The listing builds one solid part. Answer for the finished solid, in the listing's coordinates (mm). Face numbers are marked on the shaded views. A direction names the side the tool comes from. Give positions to 0.01 mm unless a question says otherwise; leave off trailing zeros. Write each loop counter-clockwise with the first axis right and the second up, starting at its lowest first coordinate (ties: lowest second). Pieces come first, ordered by that corner, then holes. Notation, with made-up numbers: (43.5, 28.5) -> (84.5, 28.5) arc R30 ccw to (84.5, 60.5) -> close; hole circle Ø5 at (-18, 10.5). An arc over 180 degrees is marked (long way). Put each result on its own line as item: value. Start each with the question number.
1) A cutting plane is placed at C-C (z = 3). Give the number of separate pieces and of enclosed holes in the cut face, then the cut area to 3 significant figures.
2) A cutting plane is placed at A-A (x = 4.5). Write down the section's boundary in (y, z).
3) A cutting plane is placed at B-B (x = 1.75). Write down the section's boundary in (y, z).
4) Find the intervals of material crossed by line 1 along Y through (x, z) = (4.5, 1.75); line 2 along Y through (x, z) = (5.25, 2); line 3 along Z through (x, y) = (1.25, 6), in increasing order. Write a range as from..to.
5) Flat-ended cylindrical pins translate along their axes: pin 1 Ø1.6 at (x, z) = (3, 5) entering from -Y; pin 2 Ø1 at (x, y) = (6, 3) entering from +Z. Find the tip coordinate at first contact, or state that the pin passes through.
6) For the marked faces 1 and 2, determine the directions among +Z, -Z, +X, -X, +Y, -Y from which every point of the face is accessible in a straight line to the end or side of a thin tool.
Autodesk Inventor part; units mm, degrees
ref_plane "YZ Plane" through (0, 0, 0) normal (1, 0, 0) x (0, 1, 0)
ref_plane "XZ Plane" through (0, 0, 0) normal (0, 1, 0) x (-1, 0, 0)
ref_plane "XY Plane" through (0, 0, 0) normal (0, 0, 1) x (1, 0, 0)
sketch "Skizze5" plane through (0, 0, 0) normal (1, 0, 0) x (0, 1, 0)
  line L0 (0, 0) -> (0.5, 0)
  line L1 (0.5, 0) -> (4.9737, 0.486)
  line L2 (4.9737, 0.486) -> (11.4319, -0.2498)
  line L3 (11.4319, -0.2498) -> (11.9319, -0.2498)
  line L4 (11.9319, -0.2498) -> (11.9319, 5.2288)
  line L5 (11.9319, 5.2288) -> (4.9737, 6.0216)
  line L6 (0, 3.4663) -> (0, 0)
  line L7 (0, 3.4663) -> (4.9737, 4.0066)
  line L8 (4.9737, 8.0188) -> (4.9737, 2.9641) construction
  line L9 (4.9737, 6.0216) -> (4.9737, 4.0066)
  point P0 (0, 0)
  dimension "d21" = 0.5
  dimension "d22" = 6.2
  dimension "d23" = 6.5
  dimension "d24" = 4.5
  dimension "d25" = 6.5
  dimension "d26" = 5.5
  dimension "d27" = 3.5
extrude "Extrusion3" add sketch "Skizze5" along normal blind 8
sketch "Skizze6" plane through (8, 11.4319, -0.2498) normal (0, -0.1132032, -0.9935719) x (-1, 0, 0)
  circle A0 centre (4, -3.625) radius 2.45
  line L0 (4, 1.8046) -> (4, -8.9328)
  line L1 (-1.3459, -3.625) -> (9.5603, -3.625)
  line L2 (8, -0.1234) -> (8, -7.1266)
  line L3 (8, 0.4968) -> (0, 0.4968)
  point P0 (8, -11.3867)
  point P1 (8, -3.625)
  point P2 (4, 0.4968)
  dimension "d30" = 4.9
extrude "Extrusion4" cut sketch "Skizze6" against normal through all
sketch "Skizze7" plane through (8, 4.9737, 0.486) normal (0, 0.1079994, -0.994151) x (-1, 0, 0)
  line L0 (-0.1981, -2.25) -> (9.2596, -2.25)
  line L1 (4, -0.3434) -> (4, -7.0095)
  line L2 (8, -4.9971) -> (0, -4.9971)
  line L3 (8, -4.5) -> (8, 0)
  circle A0 centre (4, -2.25) radius 1.5
  point P0 (4, -4.9971)
  point P1 (8, -2.25)
  dimension "d33" = 3
extrude "Extrusion5" cut sketch "Skizze7" against normal through all
sketch "Skizze8" plane through (0, 11.4319, -0.2498) normal (0, 0, -1) x (-1, 0, 0)
  line L0 (-8, -6.4582) -> (-8, 0)
  line L1 (-8, -10.9319) -> (-8, -6.4582)
  line L2 (-8, -11.4319) -> (-8, -10.9319)
  line L3 (0, -11.4319) -> (-8, -11.4319)
  line L4 (0, -11.4319) -> (0, -10.9319)
  line L5 (0, -10.9319) -> (0, -6.4582)
  line L6 (0, -6.4582) -> (0, 0)
  line L7 (0, 0) -> (0, 0.5)
  line L8 (0, 0.5) -> (-8, 0.5)
  line L9 (-8, 0) -> (-8, 0.5)
extrude "Extrusion6" add sketch "Skizze8" against normal blind 0.75
sketch "Skizze9" plane through (0, 4.9737, 6.0216) normal (0, 0.1132032, 0.9935719) x (1, 0, 0)
  circle A0 centre (4, 3.5016) radius 2.45
  point P0 (0, -4.26)
extrude "Extrusion7" cut sketch "Skizze9" against normal through all
sketch "Skizze10" plane through (0, 0, 3.4663) normal (0, -0.1079994, 0.994151) x (1, 0, 0)
  circle A0 centre (4, 2.3727) radius 1.5
  point P0 (0, -0.3744)
extrude "Extrusion8" cut sketch "Skizze10" against normal through all
chamfer "Fase2" distance 0.5 angle 45 7 edges at (8, 5.9659, -0.2498) (4, 11.9319, -0.2498) (8, 11.9319, 2.4895) (0, 5.9659, -0.2498) (0, 11.9319, 2.4895) (8, 4.9737, 5.0141) (0, 4.9737, 5.0141)
properties part number "led_holder_v11"
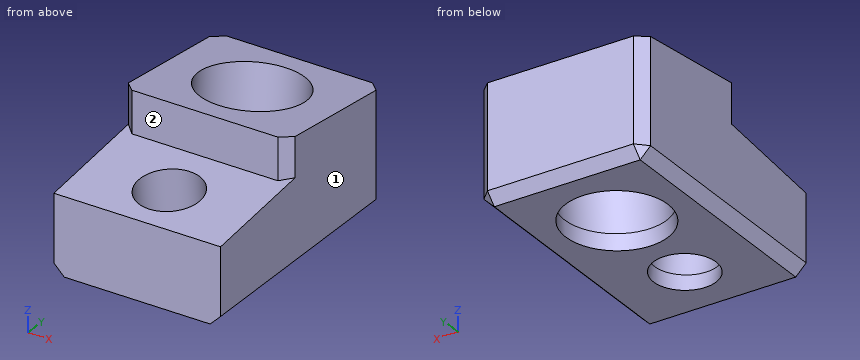
Reply:
1. separate pieces: 1
1. enclosed holes: 2
1. area: 69.1 mm2
2. outline: (0, -0.25) -> (1.37, -0.25) -> (0.95, 3.57) -> (0, 3.47) -> close; (3.76, 3.88) -> (4.21, -0.25) -> (5.37, -0.25) -> (6.07, 5.9) -> (4.97, 6.02) -> (4.97, 4.01) -> close; (10.2, -0.25) -> (11.43, -0.25) -> (11.93, 0.25) -> (11.93, 5.23) -> (10.84, 5.35) -> close
3. outline: (0, -0.25) -> (6.81, -0.25) -> (7.49, 5.73) -> (4.97, 6.02) -> (4.97, 4.01) -> (0, 3.47) -> close; (8.76, -0.25) -> (11.43, -0.25) -> (11.93, 0.25) -> (11.93, 5.23) -> (9.42, 5.52) -> close
4. line 1: y = 0..1.15, 4..5.6, 10.43..11.93
4. line 2: y = 0..1.71, 3.38..5.92, 10.16..11.93
4. line 3: z = -0.25..5.9
5. pin 1: stops at y = 4.97
5. pin 2: stops at z = 3.85
6. face 1: +Z, -Z, +X, +Y, -Y
6. face 2: +Z, +X, -X, -Y
